Check sheet for the modelled part. Datum: model origin and axes. Units: mm. Face numbers are marked on the shaded views. A direction names the side the tool comes from. Give positions to 0.01 mm unless a question says otherwise; leave off trailing zeros. Write each loop counter-clockwise with the first axis right and the second up, starting at its lowest first coordinate (ties: lowest second). Pieces come first, ordered by that corner, then holes.
from build123d import *

# Parameters (mm, degrees)
F0_W     = 129.5
F0_H     = 96.5
F0_W_2   = 123.5
F0_H_2   = 90.5
F1_DEPTH = 10
F2_R     = 2
F3_W     = 129.5
F3_H     = 96.5
F4_DEPTH = 3
F5_R     = 5
F6_SIZE  = 0.5


with BuildPart() as f1:
    # F0 (on Top) → F1 (new body)
    with BuildSketch(Plane.XY):
        with Locations((-61.75, -60.5614758432)):
            Rectangle(F0_W, F0_H)
        with Locations((-61.75, -60.5614758432)):
            Rectangle(F0_W_2, F0_H_2, mode=Mode.SUBTRACT)
    extrude(amount=F1_DEPTH)

    # F2
    f2_edges = [f1.edges().sort_by_distance(p)[0] for p in [
        (-123.5, -105.811476, 5),
        (-61.75, -105.811476, 10),
        (-61.75, -15.311476, 10),
        (-123.5, -60.561476, 10),
        (0, -15.311476, 5),
        (0, -60.561476, 10),
        (0, -105.811476, 5),
        (-123.5, -15.311476, 5),
    ]]
    fillet(f2_edges, radius=F2_R)

    # F3 (on face) → F4 (join)
    with BuildSketch(Plane(origin=(0, 0, 0), x_dir=(1, 0, 0), z_dir=(0, 0, -1))):
        with Locations((-61.75, 60.5614758432)):
            Rectangle(F3_W, F3_H)
    extrude(amount=F4_DEPTH)

    # F5
    f5_edges = [f1.edges().sort_by_distance(p)[0] for p in [
        (-126.5, -108.811476, 3.5),
        (3, -108.811476, 3.5),
        (3, -12.311476, 3.5),
        (-126.5, -12.311476, 3.5),
    ]]
    fillet(f5_edges, radius=F5_R)

    # F6
    f6_edges = [f1.edges().sort_by_distance(p)[0] for p in [
        (-125.035534, -107.34701, -3),
        (-61.75, -108.811476, -3),
        (-126.5, -60.561476, -3),
        (1.535534, -107.34701, -3),
        (3, -60.561476, -3),
        (-125.035534, -13.775942, -3),
        (-61.75, -12.311476, -3),
        (1.535534, -13.775942, -3),
    ]]
    chamfer(f6_edges, length=F6_SIZE)


solid = f1.part
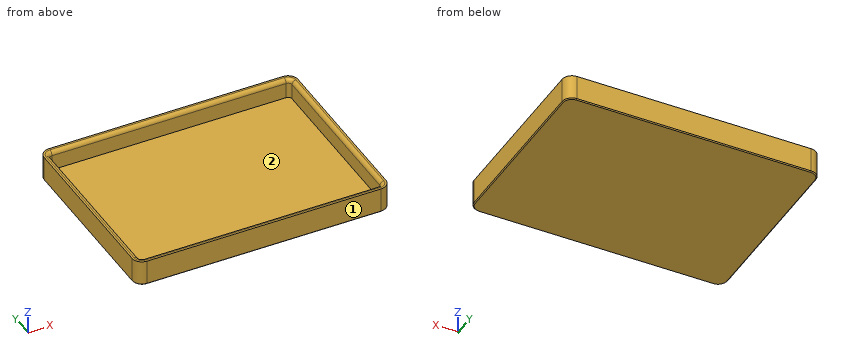
1) Sectioned sample at C-C on x = -8.5. Record the boundary of the cut face in (y, z).
2) Access from +Z, -Z, +X, -X, +Y, -Y to the whole of each face (thin tool, end or side, straight path). Record for the marked faces 1 and 2.
3) Sectioned sample at A-A on z = 5. Record the boundary of the cut face in (x, y).
4) Scan lines: L1, parallel to Y at x = -99.5, z = 4.25; L2, parallel to X at y = -41, z = 4.75; L3, parallel to Z at x = -42, y = -87.5. Record each from-to range of solid material in increasing order.
5) Sectioned sample at B-B on y = -79. Record the boundary of the cut face in (x, z).
6) Gauge pin test, flat end, axial feed: pin 1 (10 mm diameter, centred on x = -102.5, y = -40.5, fed in from +Z). Record the tip position at first contact, or that the pin passes through.
Answers below:
1. outline: (-108.81, -2.5) - (-108.31, -3) - (-12.81, -3) - (-12.31, -2.5) - (-12.31, 10) - (-13.31, 10) arc R2 ccw to (-15.31, 8) - (-15.31, 0) - (-105.81, 0) - (-105.81, 8) arc R2 ccw to (-107.81, 10) - (-108.81, 10) - close
2. face 1: +Z, -Z, +X, -X, -Y
2. face 2: +Z
3. outline: (-126.5, -103.81) arc R5 ccw to (-121.5, -108.81) - (-2, -108.81) arc R5 ccw to (3, -103.81) - (3, -17.31) arc R5 ccw to (-2, -12.31) - (-121.5, -12.31) arc R5 ccw to (-126.5, -17.31) - close; hole (-123.5, -103.81) arc R2 ccw to (-121.5, -105.81) - (-2, -105.81) arc R2 ccw to (0, -103.81) - (0, -17.31) arc R2 ccw to (-2, -15.31) - (-121.5, -15.31) arc R2 ccw to (-123.5, -17.31) - close
4. L1: y = -108.81 to -105.81, -15.31 to -12.31
4. L2: x = -126.5 to -123.5, 0 to 3
4. L3: z = -3 to 0
5. outline: (-126.5, -2.5) - (-126, -3) - (2.5, -3) - (3, -2.5) - (3, 10) - (2, 10) arc R2 ccw to (0, 8) - (0, 0) - (-123.5, 0) - (-123.5, 8) arc R2 ccw to (-125.5, 10) - (-126.5, 10) - close
6. pin 1: stops at z = 0
